Build history of the part. All positions in model axes, mm. Coordinates: 2 decimals unless noted, no trailing zeros. Write each loop counter-clockwise with the first axis right and the second up, starting at its lowest first coordinate (ties: lowest second). Pieces come first, ordered by that corner, then holes.
```python
from build123d import *

# Parameters (mm, degrees)
F1_DEPTH = 2
F2_W     = 20
F2_H     = 12
F3_DEPTH = 5
F4_R     = 1


with BuildPart() as f1:
    # F0 (on Top) → F1 (new body)
    with BuildSketch(Plane.XY):
        Polygon((-40, 0), (0, 0), (40, 0), (40, 30), (10, 30), (10, 40), (-40, 40), align=None)
    extrude(amount=F1_DEPTH)

    # F2 (on face) → F3 (cut)
    with BuildSketch(Plane.XY.offset(2)):
        with Locations((15, 19)):
            Rectangle(F2_W, F2_H)
    extrude(amount=-F3_DEPTH, mode=Mode.SUBTRACT)

    # F4
    f4_edges = [f1.edges().sort_by_distance(p)[0] for p in [
        (-15, 40, 2),
        (-40, 20, 2),
        (0, 0, 2),
        (40, 15, 2),
        (25, 30, 2),
        (10, 35, 2),
        (15, 25, 2),
        (5, 19, 2),
        (15, 13, 2),
        (25, 19, 2),
    ]]
    fillet(f4_edges, radius=F4_R)


solid = f1.part
```
1. Flat gauge pin, fed straight in: pin 1 (0.8 mm diameter, centred on x = 15.5, z = 0.5, fed in from +Y). Where does the tip first touch, or does it go through?
Computed values:
pin 1: stops at y = 30
2. Saw through at B-B on z = 0.5. List the corners of the cut face in (x, y), plus the area to 3 significant figures.
Computed values:
outline: (-40, 0) - (40, 0) - (40, 30) - (10, 30) - (10, 40) - (-40, 40) - close; hole (5, 13) - (25, 13) - (25, 25) - (5, 25) - close
area: 2,660 mm2
3. Saw through at A-A on y = 20.5. List the corners of the cut face in (x, z), plus the area to 3 significant figures.
Computed values:
outline: (-40, 0) - (5, 0) - (5, 1) arc R1 ccw to (4, 2) - (-39, 2) arc R1 ccw to (-40, 1) - close; (25, 0) - (40, 0) - (40, 1) arc R1 ccw to (39, 2) - (26, 2) arc R1 ccw to (25, 1) - close
area: 119 mm2
4. Saw through at C-C on x = 13.5. List the corners of the cut face in (y, z), plus the area to 3 significant figures.
Computed values:
outline: (0, 0) - (13, 0) - (13, 1) arc R1 ccw to (12, 2) - (1, 2) arc R1 ccw to (0, 1) - close; (25, 0) - (30, 0) - (30, 1) arc R1 ccw to (29, 2) - (26, 2) arc R1 ccw to (25, 1) - close
area: 35.1 mm2
5. Probe line 1 along X through (y, z) = (11, 1.05); line 2 along X through (y, z) = (19.5, 1.85); line 3 along X through (y, z) = (35.5, 0.9). List the from-to ranges inside material, lowest first.
Computed values:
line 1: x = -40 to 40
line 2: x = -39.53 to 4.53, 25.47 to 39.53
line 3: x = -40 to 10
6. Saw through at D-D on x = 28. List the corners of the cut face in (y, z), plus the area to 3 significant figures.
Computed values:
outline: (0, 0) - (30, 0) - (30, 1) arc R1 ccw to (29, 2) - (1, 2) arc R1 ccw to (0, 1) - close
area: 59.6 mm2
